```python
from build123d import *

# Parameters (mm, degrees)
SKETCH1_R                = 9.525
EXTRUDE1_DEPTH           = 7
F_5_16_24_TAPPED_HOLE1_D = 6.9088
SKETCH3_OUTSIDE_W        = 26.618
SKETCH3_OUTSIDE_H        = 26.618
SKETCH3_OUTSIDE_R        = 7.925
EXTRUDE3_DEPTH           = 3


with BuildPart() as part:
    # Sketch1 → Extrude1 (new body)
    with BuildSketch(Plane(origin=(0, 0, 0), x_dir=(1, 0, 0), z_dir=(0, 1, 0))):
        Circle(SKETCH1_R)
    extrude(amount=EXTRUDE1_DEPTH)

    # 5/16-24 Tapped Hole1 (through all)
    with Locations(Plane(origin=(0, 0, 0), x_dir=(-1, 0, 0), z_dir=(0, -1, 0))):
        with Locations((0, 0)):
            Hole(F_5_16_24_TAPPED_HOLE1_D / 2)

    # Sketch3 outside → Extrude3 (cut)
    with BuildSketch(Plane(origin=(0, 7, 0), x_dir=(1, 0, 0), z_dir=(0, 1, 0))):
        Rectangle(SKETCH3_OUTSIDE_W, SKETCH3_OUTSIDE_H)
        Circle(SKETCH3_OUTSIDE_R, mode=Mode.SUBTRACT)
    extrude(amount=-EXTRUDE3_DEPTH, mode=Mode.SUBTRACT)

    # Sketch6 → Cut-Revolve1 (revolve, cut)
    with BuildSketch(Plane.XY):
        Polygon((-9.525, 2.8), (-7, 0), (-7, -3.811390031), (-11.858524977, -3.811390031), (-11.858524977, 2.8), align=None)
    revolve(axis=Axis((0, 0, 0), (0, 1, 0)), mode=Mode.SUBTRACT)


solid = part.part
```
Check sheet for the modelled part. Datum: model origin and axes. Units: mm. A direction names the side the tool comes from. Give positions to 0.01 mm unless a question says otherwise; leave off trailing zeros. Order: outer loops, then holes, each group sorted by start corner. A loop starts at its lowest first (then second) coordinate and runs counter-clockwise, first axis right, second up. Notation, with made-up numbers: M 37.5,68 L 95.5,68 A28 ccw 95.5,97 Z; hole C 11,11.25 d11. An arc over 180 degrees is marked long. Answer in a Markdown table with one row per item.
1) Cross-section at A-A, the plane x = 0. Enter the section's corners in (y, z) (3 decimals), plus the area to 3 significant figures.
Filled sheet:
| item | result |
|---|---|
| outline | M 0,-7 L 2.8,-9.525 L 4,-9.525 L 4,-7.925 L 7,-7.925 L 7,-3.454 L 0,-3.454 Z; M 0,3.454 L 7,3.454 L 7,7.925 L 4,7.925 L 4,9.525 L 2.8,9.525 L 0,7 Z |
| area | 68.3 mm2 |
2) Gauge pin test, flat ends, axial feed: P1, Ø1, axis at y = 1, z = 6, coming from the -X side; P2, Ø1.5, axis at y = 4.5, z = -5.5, coming from the -X side; P3, Ø4, axis at x = -6.5, y = 1.5, coming from the +Z side; P4, Ø4, axis at x = 0, z = 0, coming from the +Y side. Record the tip position at first contact, or that the pin passes through.
Filled sheet:
| item | result |
|---|---|
| P1 | stops at x = -5.98 |
| P2 | stops at x = -8.14 |
| P3 | stops at z = 8.12 |
| P4 | passes through |
3) Access from +Z, -Z, +X, -X, +Y, -Y to the whole of each face (thin tool, end or side, straight path). Record for faces 4 (the conical face through (5.652, 0.136, -4.334)), 5 (the flat face through (-2, 4, -8)).
Filled sheet:
| item | result |
|---|---|
| face 4 | -Y |
| face 5 | +Y |
4) Cross-section at C-C, the plane y = 1.75. Enter the section's corners in (x, z).
Filled sheet:
| item | result |
|---|---|
| outline | C 0,0 d17.16; hole C 0,0 d6.91 |
5) Cross-section at B-B, the plane z = 0. Enter the section's corners in (x, y) (3 decimals).
Filled sheet:
| item | result |
|---|---|
| outline | M -9.525,2.8 L -7,0 L -3.454,0 L -3.454,7 L -7.925,7 L -7.925,4 L -9.525,4 Z; M 3.454,0 L 7,0 L 9.525,2.8 L 9.525,4 L 7.925,4 L 7.925,7 L 3.454,7 Z |
6) Thickness scan on L1, parallel to Z at x = 0, y = 5 (3 decimals); L2, parallel to X at y = 6.75, z = -2.5. Record the ranges inside material, lowest first. Write a range as [from, to].
Filled sheet:
| item | result |
|---|---|
| L1 | z = [-7.925, -3.454], [3.454, 7.925] |
| L2 | x = [-7.52, -2.38], [2.38, 7.52] |
7) Release check for a two-part mould opening along X. For faces 1 (the flat face through (-3, 0, -2)), 2 (the cylindrical face through (-7.559, 3.392, 5.796)), 3 (the cylindrical face through (-0.45, 3.549, -3.425)) record: +X half, -X half, draft (parallel to the pull), parting line (faces both ways), or undercut.
Filled sheet:
| item | result |
|---|---|
| face 1 | draft |
| face 2 | parting line |
| face 3 | undercut |
